```python
from build123d import *

# Parameters (mm, degrees)
BASE_MOUNTED_START            = 27
SKETCH1_W                     = 4
SKETCH1_H                     = 6.4
BASE_MOUNTED_STOP_BLOCK_DEPTH = 30
SKETCH2_R                     = 2.56
M6_TAP_CORE_DEPTH             = 4


with BuildPart() as part:
    # Sketch1 → Base-mounted stop block (new body)
    with BuildSketch(Plane.XY.offset(BASE_MOUNTED_START)):
        with Locations((2, 80.8)):
            Rectangle(SKETCH1_W, SKETCH1_H)
    extrude(amount=BASE_MOUNTED_STOP_BLOCK_DEPTH)

    # Sketch2 → M6 tap core (cut)
    with BuildSketch(Plane(origin=(0, 0, 0), x_dir=(0, 0, -1), z_dir=(1, 0, 0))):
        with Locations((-50, 80.8)):
            Circle(SKETCH2_R)
    extrude(amount=M6_TAP_CORE_DEPTH, mode=Mode.SUBTRACT)


solid = part.part
```
Here's how the part is built. I have some questions about the finished solid (model axes, mm). Round coordinates to 2 decimals unless told otherwise and drop trailing zeros. Order: outer loops, then holes, each group sorted by start corner. A loop starts at its lowest first (then second) coordinate and runs counter-clockwise, first axis right, second up. Notation, with made-up numbers: (60, 52.5) -> (92, 52.5) arc R28 cw to (92, 74.5) -> close; hole circle Ø1 at (38.25, 25.25). An arc over 180 degrees is marked (long way). Use a Markdown table: item, result. Add a question column.
(1) If we mould it in two halves opening along Z, with no side actions, what happens to faces 1 (the face through (2, 81, 27)), 2 (the face through (4, 81, 42)), 3 (the face through (2, 81, 57)), 4 (the face through (1.97, 78.53, 48.82))? For each: released by +Z, released by -Z, zero draft, split by the parting line, or undercut.
(2) Suppose I cut it at B-B, the plane z = 50. Please give me the cut outline in (x, y), and give its area (3 significant figures).
(3) I need wall thicknesses on line 1 along Y through (x, z) = (0.95, 50); line 2 along Z through (x, y) = (1.25, 80.25); line 3 along Z through (x, y) = (2.2, 80). Which ranges of each line are inside material? Lowest first, please.
(4) Suppose I cut it at C-C, the plane x = 2.8. Please give me the cut outline in (y, z).
(5) Suppose I cut it at A-A, the plane y = 80.8. Please give me the cut outline in (x, z), and give its area (3 significant figures).
Verdict:
| question | item | result |
|---|---|---|
| 1 | face 1 | released by -Z |
| 1 | face 2 | zero draft |
| 1 | face 3 | released by +Z |
| 1 | face 4 | undercut |
| 2 | outline | (0, 77.6) -> (4, 77.6) -> (4, 78.24) -> (0, 78.24) -> close; (0, 83.36) -> (4, 83.36) -> (4, 84) -> (0, 84) -> close |
| 2 | area | 5.12 mm2 |
| 3 | line 1 | 77.6 to 78.24, 83.36 to 84 |
| 3 | line 2 | 27 to 47.5, 52.5 to 57 |
| 3 | line 3 | 27 to 47.57, 52.43 to 57 |
| 4 | outline | (77.6, 27) -> (84, 27) -> (84, 57) -> (77.6, 57) -> close; hole circle Ø5.12 at (80.8, 50) |
| 5 | outline | (0, 27) -> (4, 27) -> (4, 47.44) -> (0, 47.44) -> close; (0, 52.56) -> (4, 52.56) -> (4, 57) -> (0, 57) -> close |
| 5 | area | 99.5 mm2 |
